```python
from build123d import *

# Parameters (mm, degrees)
EXTRUDE_1_DEPTH = 1.5
SKETCH_3_R      = 16.2
EXTRUDE_2_DEPTH = 0.1
EXTRUDE_3_DEPTH = 0.3
FILLET_1_R      = 0.5


with BuildPart() as part:
    # 草图1 → 凸台-拉伸1 (new body)
    with BuildSketch(Plane(origin=(0, 0, 0), x_dir=(1, 0, 0), z_dir=(0, 1, 0))):
        with BuildLine():
            Line((20.3, 6.75), (20.3, -6.75))
            Line((20.3, -6.75), (15.17728566, -9.3))
            ThreePointArc((15.17728566, -9.3), (-17.8, 0), (15.17728566, 9.3))
            Line((15.17728566, 9.3), (20.3, 6.75))
        make_face()
    extrude(amount=EXTRUDE_1_DEPTH)

    # 草图3 → 凸台-拉伸2 (add)
    with BuildSketch(Plane(origin=(0, 1.5, 0), x_dir=(1, 0, 0), z_dir=(0, 1, 0))):
        Circle(SKETCH_3_R)
    extrude(amount=EXTRUDE_2_DEPTH)

    # 草图4 → 凸台-拉伸3 (add)
    with BuildSketch(Plane.XZ):
        Polygon((20.8, -6.24), (20.8, 5.7), (10.06, 5.7), (10.06, -5.7), (13.26, -5.7), (13.8, -6.24), align=None)
        with BuildLine():
            add(Edge.make_bspline(
                [(10.818486802, -4.395328042), (10.805172896, -4.40810149), (10.777735498, -4.434425106), (10.731585338, -4.471001471), (10.680718947, -4.50727864), (10.644265505, -4.529889796), (10.625504346, -4.541526873)],
                knots=[0, 0, 0, 0, 5.5324e-05, 0.000114012, 0.000176454, 0.000242669, 0.000242669, 0.000242669, 0.000242669], degree=3))
            Line((10.625504346, -4.541526873), (10.625504346, -4.430415762))
            add(Edge.make_bspline(
                [(10.625504346, -4.430415762), (10.637511845, -4.422097374), (10.661358973, -4.405576894), (10.695199347, -4.378706463), (10.727916327, -4.35134661), (10.758520561, -4.322379824), (10.787985268, -4.292793589), (10.815334495, -4.261758783), (10.841379972, -4.22987118), (10.857300173, -4.207631606), (10.865270428, -4.196497633)],
                knots=[0, 0, 0, 0, 4.381e-05, 8.7008e-05, 0.000129577, 0.000171717, 0.000213376, 0.0002548, 0.000295763, 0.000336832, 0.000336832, 0.000336832, 0.000336832], degree=3))
            Line((10.865270428, -4.196497633), (10.935445867, -4.196497633))
            Line((10.935445867, -4.196497633), (10.935445867, -5.202345586))
            Line((10.935445867, -5.202345586), (10.818486802, -5.202345586))
            Line((10.818486802, -5.202345586), (10.818486802, -4.395328042))
        make_face(mode=Mode.SUBTRACT)
        with BuildLine():
            add(Edge.make_bspline(
                [(10.747897656, 4.993028455), (10.734583749, 4.980255007), (10.707146352, 4.953931392), (10.660996192, 4.917355027), (10.610129801, 4.881077858), (10.573676359, 4.858466702), (10.5549152, 4.846829625)],
                knots=[0, 0, 0, 0, 5.5324e-05, 0.000114012, 0.000176454, 0.000242669, 0.000242669, 0.000242669, 0.000242669], degree=3))
            Line((10.5549152, 4.846829625), (10.5549152, 4.957940736))
            add(Edge.make_bspline(
                [(10.5549152, 4.957940736), (10.566922699, 4.966259124), (10.590769826, 4.982779604), (10.6246102, 5.009650034), (10.65732718, 5.037009887), (10.687931415, 5.065976673), (10.717396122, 5.095562908), (10.744745348, 5.126597715), (10.770790825, 5.158485318), (10.786711026, 5.180724892), (10.794681281, 5.191858864)],
                knots=[0, 0, 0, 0, 4.381e-05, 8.7008e-05, 0.000129577, 0.000171717, 0.000213376, 0.0002548, 0.000295763, 0.000336832, 0.000336832, 0.000336832, 0.000336832], degree=3))
            Line((10.794681281, 5.191858864), (10.86485672, 5.191858864))
            Line((10.86485672, 5.191858864), (10.86485672, 4.186010911))
            Line((10.86485672, 4.186010911), (10.747897656, 4.186010911))
            Line((10.747897656, 4.186010911), (10.747897656, 4.993028455))
        make_face(mode=Mode.SUBTRACT)
        with BuildLine():
            add(Edge.make_bspline(
                [(11.239125726, 4.209402724), (11.239833141, 4.216646412), (11.241239164, 4.23104361), (11.246176296, 4.252223765), (11.253123203, 4.272903106), (11.262262649, 4.29307236), (11.273547522, 4.312739702), (11.287428195, 4.331488732), (11.302928415, 4.350145808), (11.321465332, 4.367779976), (11.341452247, 4.386542756), (11.362154394, 4.408019092), (11.384577692, 4.431466047), (11.407813575, 4.457882847), (11.432843118, 4.486319526), (11.458703548, 4.517616287), (11.486012518, 4.551174546), (11.514003658, 4.586370362), (11.541434011, 4.621720239), (11.56671184, 4.65597954), (11.589699984, 4.687968259), (11.610212924, 4.717799327), (11.627704069, 4.745816407), (11.642893445, 4.771584725), (11.655854012, 4.795057685), (11.668787399, 4.823092213), (11.680993939, 4.855423395), (11.690565178, 4.892152564), (11.694914493, 4.926144912), (11.693204675, 4.957381602), (11.686490374, 4.98588729), (11.674759334, 5.011748614), (11.658296591, 5.035057433), (11.637248958, 5.054942362), (11.613257207, 5.071313574), (11.586558607, 5.082313299), (11.557991357, 5.087872292), (11.528104736, 5.087369351), (11.497980127, 5.082013566), (11.467969579, 5.072704256), (11.439039112, 5.058289936), (11.410696566, 5.040307531), (11.384436934, 5.017140759), (11.36135616, 4.988611831), (11.341721738, 4.954866078), (11.331926076, 4.929936265), (11.326845024, 4.917005063)],
                knots=[0, 0, 0, 0, 2.1814e-05, 4.3357e-05, 6.5069e-05, 8.7171e-05, 0.000109684, 0.000132949, 0.000157077, 0.000182347, 0.000209615, 0.000239329, 0.00027181, 0.000306939, 0.000344857, 0.000385456, 0.00042872, 0.000474656, 0.000520361, 0.000562944, 0.000602373, 0.000638538, 0.000671529, 0.000701432, 0.000728277, 0.000751921, 0.000794003, 0.000831773, 0.00086557, 0.000896375, 0.00092511, 0.00095293, 0.000981054, 0.00101016, 0.001039355, 0.001067712, 0.001096172, 0.001126062, 0.001156827, 0.001187721, 0.001219978, 0.001253501, 0.00128818, 0.001324511, 0.001363144, 0.00140478, 0.00140478, 0.00140478, 0.00140478], degree=3))
            Line((11.326845024, 4.917005063), (11.215733913, 4.934548923))
            add(Edge.make_bspline(
                [(11.215733913, 4.934548923), (11.219656813, 4.945425545), (11.227289073, 4.966586728), (11.240431556, 4.996719226), (11.254008051, 5.024768665), (11.268391205, 5.050549193), (11.283893055, 5.073876788), (11.300137608, 5.094978241), (11.317197246, 5.113850725), (11.335137556, 5.130472165), (11.35389693, 5.145124772), (11.373604192, 5.157831984), (11.394013956, 5.168932074), (11.415206508, 5.178352557), (11.43722761, 5.185944542), (11.460175176, 5.191465532), (11.483814494, 5.195748716), (11.499956502, 5.19704853), (11.508131574, 5.197706818)],
                knots=[0, 0, 0, 0, 3.4679e-05, 6.747e-05, 9.8564e-05, 0.000128143, 0.000155956, 0.000182513, 0.000207966, 0.000232182, 0.000255794, 0.000279284, 0.000302447, 0.000325428, 0.000348785, 0.000372214, 0.000396178, 0.000420768, 0.000420768, 0.000420768, 0.000420768], degree=3))
            add(Edge.make_bspline(
                [(11.508131574, 5.197706818), (11.517654805, 5.198470616), (11.536175647, 5.199956055), (11.563321528, 5.200235741), (11.588939793, 5.198463956), (11.613483722, 5.195099015), (11.637461864, 5.189150579), (11.661491911, 5.180373219), (11.685801114, 5.168509643), (11.710349938, 5.153958828), (11.73441354, 5.136146543), (11.756199385, 5.11374856), (11.775424492, 5.087198528), (11.792601639, 5.05716399), (11.806466377, 5.023396102), (11.814804628, 4.985783772), (11.817862258, 4.944983333), (11.816182176, 4.908994618), (11.812089602, 4.878541375), (11.806355457, 4.854202585), (11.798091587, 4.828865854), (11.788361792, 4.802138754), (11.775441683, 4.774655097), (11.760899169, 4.745824926), (11.74350862, 4.716170927), (11.727726825, 4.690551343), (11.713428345, 4.669220128), (11.70145212, 4.651813704), (11.688368763, 4.633233154), (11.673683781, 4.613773904), (11.658174582, 4.592989779), (11.641491734, 4.571060318), (11.623490026, 4.548175641), (11.604377689, 4.524045702), (11.584068424, 4.498734851), (11.562470569, 4.472389765), (11.539590091, 4.445069691), (11.51578304, 4.416404416), (11.490759524, 4.386634205), (11.46450038, 4.355787108), (11.436918885, 4.324002126), (11.418239887, 4.302325786), (11.408716369, 4.291274069)],
                knots=[0, 0, 0, 0, 2.8656e-05, 5.5731e-05, 8.1347e-05, 0.000105638, 0.000129959, 0.000155311, 0.000182241, 0.000210992, 0.000240838, 0.000271776, 0.00030431, 0.000338939, 0.000375378, 0.000413366, 0.000453999, 0.000497793, 0.000521195, 0.000546098, 0.000572677, 0.000601119, 0.000631359, 0.000663713, 0.000697965, 0.000734447, 0.00075397, 0.000774997, 0.000797834, 0.000822135, 0.000848126, 0.000875634, 0.000904794, 0.000935474, 0.000967981, 0.001002147, 0.001037671, 0.001074887, 0.001113934, 0.001154341, 0.001196417, 0.001240183, 0.001240183, 0.001240183, 0.001240183], degree=3))
            Line((11.408716369, 4.291274069), (11.829769001, 4.291274069))
            Line((11.829769001, 4.291274069), (11.829769001, 4.186010911))
            Line((11.829769001, 4.186010911), (11.239125726, 4.186010911))
            Line((11.239125726, 4.186010911), (11.239125726, 4.209402724))
        make_face(mode=Mode.SUBTRACT)
    extrude(amount=EXTRUDE_3_DEPTH)

    # 圆角1
    fillet_1_edges = [part.edges().sort_by_distance(p)[0] for p in [
        (10.06, -0.15, -5.7),
        (10.06, -0.15, 5.7),
        (20.8, -0.15, 5.7),
        (20.8, -0.15, -6.24),
    ]]
    fillet(fillet_1_edges, radius=FILLET_1_R)


solid = part.part
```
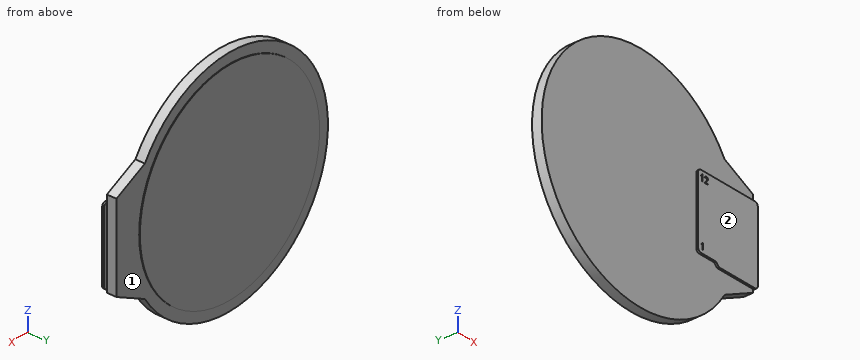
Could you check a few things on this model? Use its own coordinates, in mm. Face numbers are marked on the shaded views. A direction names the side the tool comes from. Coordinates: 2 decimals unless noted, no trailing zeros. Order: outer loops, then holes, each group sorted by start corner. A loop starts at its lowest first (then second) coordinate and runs counter-clockwise, first axis right, second up. Notation, with made-up numbers: M 23,-38.5 L 37,-38.5 A14 cw 37,-24.5 Z; hole C 50,-38 d8. An arc over 180 degrees is marked long. Use a Markdown table: item, result. Add a question column.
Q1. Which directions (+Z, -Z, +X, -X, +Y, -Y) give clear straight access to the entire face, cutting with the end or side of a thin tool? Please do the marked faces 1 and 2.
Q2. I want a section at B-B on z = -2.5. List the corners of the cut face in (x, y) for me.
Q3. I want a section at C-C on y = 1. List the corners of the cut face in (x, z) for me, then the cut area to 3 significant figures.
Q4. I want a section at D-D on z = 12.5. List the corners of the cut face in (x, y) for me, then the cut area to 3 significant figures.
Q5. I'm going to push a flat-ended pin straight in: pin 1 (1 mm diameter, centred on x = -1, z = 11, fed in from -Y). Where does the tip first touch, or does it pass through?
Q6. If I drill on L1, parallel to Y at x = -16, z = 3.5; L2, parallel to Y at x = 18, z = 5.5; L3, parallel to X at y = -0.1, z = 0, over which ranges is the centre line in solid material (lowest first)?
Q7. I want a section at A-A on x = 0. List the corners of the cut face in (y, z) for me, then the cut area to 3 significant figures.
Checked values:
| question | item | result |
|---|---|---|
| 1 | face 1 | +Y |
| 1 | face 2 | +Z, -Z, +X, -X, -Y |
| 2 | outline | M -17.62,0 L 10.06,0 L 10.06,-0.3 L 20.8,-0.3 L 20.8,0 L 20.3,0 L 20.3,1.5 L 16.01,1.5 L 16.01,1.6 L -16.01,1.6 L -16.01,1.5 L -17.62,1.5 Z |
| 3 | outline | M 15.18,-9.3 L 20.3,-6.75 L 20.3,6.75 L 15.18,9.3 A17.8 ccw long Z |
| 3 | area | 1,040 mm² |
| 4 | outline | M -12.67,0 L 12.67,0 L 12.67,1.5 L 10.3,1.5 L 10.3,1.6 L -10.3,1.6 L -10.3,1.5 L -12.67,1.5 Z |
| 4 | area | 40.1 mm² |
| 5 | pin 1 | y = 0 |
| 6 | L1 | 0 to 1.5 |
| 6 | L2 | -0.3 to 1.5 |
| 6 | L3 | 10.06 to 20.8 |
| 7 | outline | M 0,-17.8 L 1.5,-17.8 L 1.5,-16.2 L 1.6,-16.2 L 1.6,16.2 L 1.5,16.2 L 1.5,17.8 L 0,17.8 Z |
| 7 | area | 56.6 mm² |
